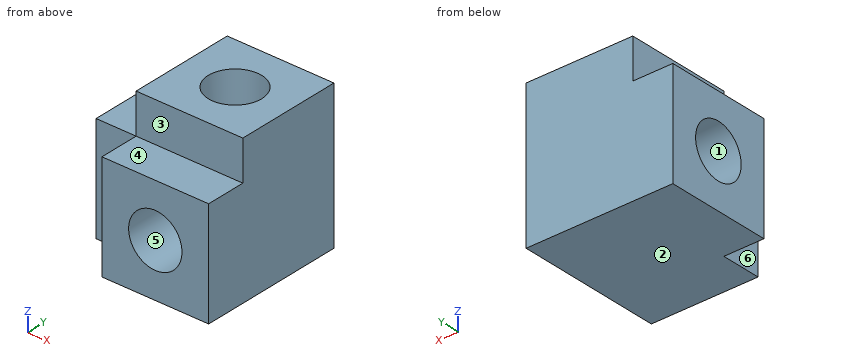
```python
from build123d import *

# Parameters (mm, degrees)
ESQUISSE2_W             = 80
ESQUISSE2_H             = 80
BOSS_EXTRU_1_DEPTH      = 80
ESQUISSE5_W             = 80
ESQUISSE5_H             = 80
BOSS_EXTRU_2_DEPTH      = 30
ESQUISSE6_W             = 80
ESQUISSE6_H             = 80
BOSS_EXTRU_3_DEPTH      = 30
ESQUISSE7_W             = 80
ESQUISSE7_H             = 80
BOSS_EXTRU_4_DEPTH      = 30
ESQUISSE8_R             = 20
ENL_V_MAT_EXTRU_1_DEPTH = 45
ESQUISSE9_R             = 20
ENL_V_MAT_EXTRU_2_DEPTH = 45
ESQUISSE10_R            = 20
ENL_V_MAT_EXTRU_3_DEPTH = 45


with BuildPart() as part:
    # Esquisse2 → Boss.-Extru.1 (new body)
    with BuildSketch(Plane(origin=(0, 0, 0), x_dir=(1, 0, 0), z_dir=(0, 1, 0))):
        Rectangle(ESQUISSE2_W, ESQUISSE2_H)
    extrude(amount=BOSS_EXTRU_1_DEPTH)

    # Esquisse5 → Boss.-Extru.2 (add)
    with BuildSketch(Plane.ZY.offset(40)):
        with Locations((0, 40)):
            Rectangle(ESQUISSE5_W, ESQUISSE5_H)
    extrude(amount=BOSS_EXTRU_2_DEPTH)

    # Esquisse6 → Boss.-Extru.3 (add)
    with BuildSketch(Plane.XY.offset(40)):
        with Locations((0, 40)):
            Rectangle(ESQUISSE6_W, ESQUISSE6_H)
    extrude(amount=BOSS_EXTRU_3_DEPTH)

    # Esquisse7 → Boss.-Extru.4 (add)
    with BuildSketch(Plane.XZ):
        Rectangle(ESQUISSE7_W, ESQUISSE7_H)
    extrude(amount=BOSS_EXTRU_4_DEPTH)

    # Esquisse8 → Enlèv. mat.-Extru.1 (cut)
    with BuildSketch(Plane.ZY.offset(70)):
        with Locations((0, 40)):
            Circle(ESQUISSE8_R)
    extrude(amount=-ENL_V_MAT_EXTRU_1_DEPTH, mode=Mode.SUBTRACT)

    # Esquisse9 → Enlèv. mat.-Extru.2 (cut)
    with BuildSketch(Plane.XY.offset(70)):
        with Locations((0, 40)):
            Circle(ESQUISSE9_R)
    extrude(amount=-ENL_V_MAT_EXTRU_2_DEPTH, mode=Mode.SUBTRACT)

    # Esquisse10 → Enlèv. mat.-Extru.3 (cut)
    with BuildSketch(Plane.XZ.offset(30)):
        with Locations(Location((0, 0, 0), (0, 0, 270))):
            Circle(ESQUISSE10_R)
    extrude(amount=-ENL_V_MAT_EXTRU_3_DEPTH, mode=Mode.SUBTRACT)


solid = part.part
```
Geometry: final body of the model. Coordinates: model frame, mm. Face numbers are marked on the shaded views. A direction names the side the tool comes from. Coordinates: 2 decimals unless noted, no trailing zeros. Loops run counter-clockwise (first coordinate to the right, second up) from the corner with the lowest first, then second, coordinate; pieces in that order, holes last. Notation, with made-up numbers: (76, 14) -> (82, 14) arc R28 cw to (82, 53) -> close; hole circle Ø8 at (40.25, 27). An arc over 180 degrees is marked (long way). Use a Markdown table: item, result. Add a question column.
(1) Section query C-C, the plane x = 0. Return loops of the section in (y, z), plus the area to 3 significant figures.
(2) Line query: line 1 along Y through (x, z) = (0, 46); line 2 along Y through (x, z) = (-36.5, 0); line 3 along Z through (x, y) = (-51.5, 2.5). Output: solid intervals per line, ascending.
(3) Pin query (flat end, axial travel): pin 1 Ø9 at (y, z) = (-16, -16.5) entering from -X; pin 2 Ø3 at (x, y) = (-5.5, 39.5) entering from +Z; pin 3 Ø5 at (x, z) = (-14.5, -8) entering from -Y. Return the tip coordinate at first contact, or that it passes through.
(4) Section query A-A, the plane z = 27. Return loops of the section in (x, y), plus the area to 3 significant figures.
(5) Mould query, pull axis Y, two halves, no side actions, for the marked faces 1, 2 and 3. Classes: pulls with the +Y half, pulls with the -Y half, needs draft (parallel to the pull), parting line crosses it, or undercut.
(6) Access query for the marked faces 4, 5 and 6. Directions: +Z, -Z, +X, -X, +Y, -Y. A direction counts if a zero-diameter tool reaches every point of the face in a straight line with its end or side. Return the directions, or none.
(7) Section query D-D, the plane y = -7. Return loops of the section in (x, z).
(8) Section query B-B, the plane y = 40. Return loops of the section in (x, z), plus the area to 3 significant figures.
Answer:
| question | item | result |
|---|---|---|
| 1 | outline | (-30, -40) -> (80, -40) -> (80, 70) -> (60, 70) -> (60, 25) -> (20, 25) -> (20, 70) -> (0, 70) -> (0, 40) -> (-30, 40) -> (-30, 20) -> (15, 20) -> (15, -20) -> (-30, -20) -> close |
| 1 | area | 7,600 mm^2 |
| 2 | line 1 | y = 0 to 20, 60 to 80 |
| 2 | line 2 | y = -30 to 20, 60 to 80 |
| 2 | line 3 | z = -40 to 40 |
| 3 | pin 1 | stops at x = -40 |
| 3 | pin 2 | stops at z = 25 |
| 3 | pin 3 | stops at y = 15 |
| 4 | outline | (-70, 0) -> (-40, 0) -> (-40, -30) -> (40, -30) -> (40, 80) -> (-70, 80) -> close; hole circle Ø40 at (0, 40) |
| 4 | area | 9,940 mm^2 |
| 5 | face 1 | undercut |
| 5 | face 2 | needs draft |
| 5 | face 3 | pulls with the -Y half |
| 6 | face 4 | +Z, +X, -X, -Y |
| 6 | face 5 | -Y |
| 6 | face 6 | +Z, -Z, -X, -Y |
| 7 | outline | (-40, -40) -> (40, -40) -> (40, 40) -> (-40, 40) -> close; hole circle Ø40 at (0, 0) |
| 8 | outline | (-70, -40) -> (40, -40) -> (40, 70) -> (20, 70) -> (20, 25) -> (-20, 25) -> (-20, 70) -> (-40, 70) -> (-40, 40) -> (-70, 40) -> (-70, 20) -> (-25, 20) -> (-25, -20) -> (-70, -20) -> close |
| 8 | area | 7,600 mm^2 |
